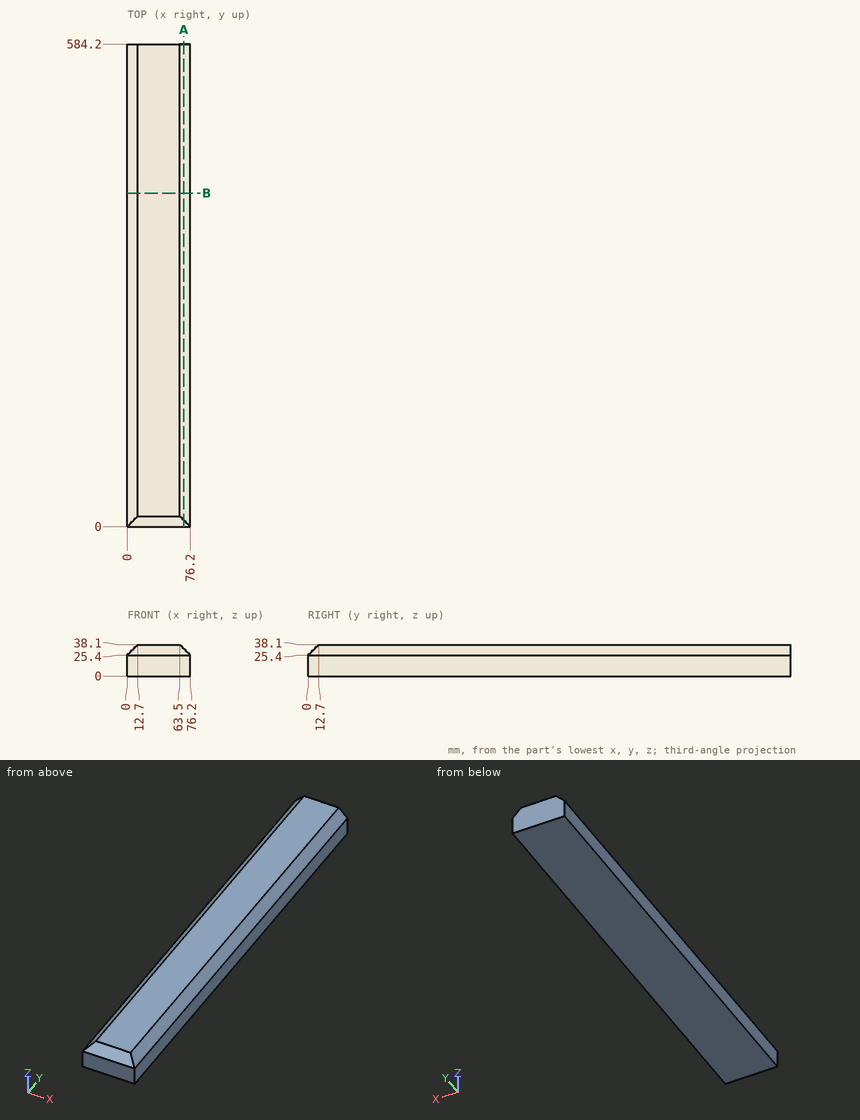
Drawing for the job (mm, zero at the part's lowest x, y, z). Give positions to 0.01 mm unless a question says otherwise; leave off trailing zeros. Order: outer loops, then holes, each group sorted by start corner. A loop starts at its lowest first (then second) coordinate and runs counter-clockwise, first axis right, second up. Notation, with made-up numbers: M -17,45 L 6,45 A12 cw 6,60 Z; hole C 5,47.25 d5. An arc over 180 degrees is marked long. Write item = value, one per line. Start each with the question number.
(1) Probe L1, parallel to Y at x = 16, z = 27; L2, parallel to X at y = 58, z = 30.5; L3, parallel to Y at x = 42.5, z = 28. List the from-to ranges inside material, lowest first. Write a range as [from, to].
(2) Pin check, flat tips, straight feed: pin 1 Ø6 at (y, z) = (298, 30) entering from +X; pin 2 Ø1 at (y, z) = (137, 32) entering from -X. Stop position of each tip, or through.
(3) Slice it at B-B on y = 403.5. Write the cut outline in (x, z).
(4) Slice it at A-A on x = 68.5. Write the cut outline in (y, z), plus the area to 3 significant figures.
Responses:
q1.L1 = [1.6, 584.2]
q1.L2 = [5.1, 71.1]
q1.L3 = [2.6, 584.2]
q2.pin_1 = 74.6
q2.pin_2 = 6.1
q3.outline = M 0,0 L 76.2,0 L 76.2,25.4 L 63.5,38.1 L 12.7,38.1 L 0,25.4 Z
q4.outline = M 0,0 L 584.2,0 L 584.2,33.1 L 7.7,33.1 L 0,25.4 Z
q4.area = 19,300 mm2
